The listing builds one solid part. Answer for the finished solid, in the listing's coordinates (mm). Face numbers are marked on the shaded views. Give positions to 0.01 mm unless a question says otherwise; leave off trailing zeros. Loops run counter-clockwise (first coordinate to the right, second up) from the corner with the lowest first, then second, coordinate; pieces in that order, holes last.
Item 1: The mould has two halves that part along Y. Classify the marked faces 1, 2, 3 and 4: pulls with the +Y half, pulls with the -Y half, needs draft (parallel to the pull), parting line crosses it, or undercut.
Item 2: Section B-B, the plane y = -11.5 is taken. Give the vertices of the cut face in (x, z) (1 decimal).
Item 3: Section D-D, the plane y = 7 is taken. Give the vertices of the cut face in (x, z) (3 decimals), and give its area (3 significant figures).
Item 4: Section C-C, the plane z = 6.25 is taken. Give the vertices of the cut face in (x, y) (3 decimals).
Item 5: Section A-A, the plane z = 3 is taken. Give the vertices of the cut face in (x, y) (3 decimals).
Item 6: This flat-tipped pin is pushed along its axis until it touches: pin 1 Ø5 at (x, y) = (-18.669, -12.319) entering from +Z (3 decimals). Where does it stop, or does it pass through?
Item 7: Consider line 1 along Y through (x, z) = (-13, 0.75) (3 decimals); line 2 along Y through (x, z) = (5, 1) (3 decimals); line 3 along Y through (x, z) = (19, 3.25) (3 decimals). Determine where each line is inside the solid, lowest interval first.
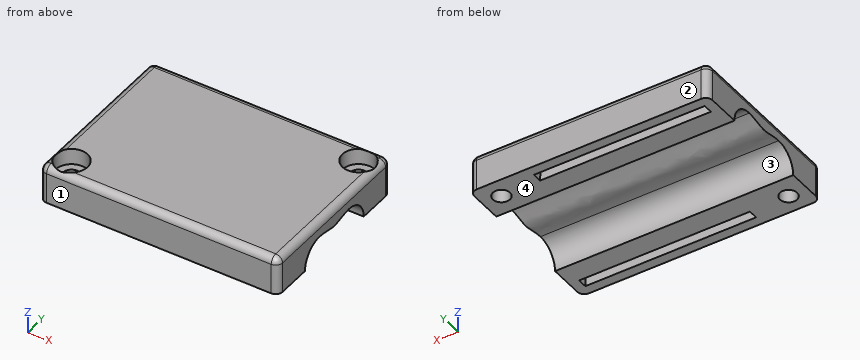
from build123d import *

# Parameters (mm, degrees)
F1_W          = 44.45
F1_H          = 31.75
F2_DEPTH      = 6.985
F4_DEPTH      = 44.45
F6_W          = 31.875
F6_H          = 1.75
F6_W_2        = 31.877
F7_DEPTH      = 2.5
F7_TAPER      = 7
F5_R          = 1.6
F8_DEPTH      = 25.4
F9_R          = 3
F9_R_2        = 1.6
F10_DEPTH     = 3
F11_T1_DEPTH  = 29.21
F11_T3_DEPTH  = 8.89
F11_T5_DEPTH  = 41.91
F11_S9_W      = 1.27
F11_S9_H      = 1.27
F11_T10_DEPTH = 1.27
F11_S15_W     = 1.27
F11_S15_H     = 1.27
F11_T16_DEPTH = 1.27
F11_S21_W     = 1.27
F11_S21_H     = 1.27
F11_T22_DEPTH = 1.27
F11_S27_W     = 1.27
F11_S27_H     = 1.27
F11_T28_DEPTH = 1.27


# Not quite as in the source:
# - a fillet or chamfer that OpenCascade refuses, or shapes differently, is made with other operations: its cross-section is extruded or revolved along the edge and cut away or added


with BuildPart() as f2:
    # F1 (on Top) → F2 (new body)
    with BuildSketch(Plane.XY):
        Rectangle(F1_W, F1_H)
    extrude(amount=F2_DEPTH)

    # F3 (on face) → F4 (cut, through all)
    with BuildSketch(Plane.YZ.offset(22.225)):
        with BuildLine():
            add(Edge.make_bspline(
                [(-4.125, 4.125), (-2.4255892558, 4.1137489608), (-0.0276085061, 2.971292738), (2.5249406681, 4.1137612248), (4.191, 4.191)],
                knots=[0, 0, 0, 0, 0.4977710734, 1, 1, 1, 1], degree=3))
            ThreePointArc((-4.125, 4.125), (-7.0418154724, 2.9168154724), (-8.25, 0))
            ThreePointArc((-8.25, 0), (-7.0418154724, -2.9168154724), (-4.125, -4.125))
            add(Edge.make_bspline(
                [(-4.125, -4.125), (-2.9335741419, -4.2006121948), (0.4172014685, -3.0581585459), (2.1438994445, -4.2006121948), (4.191, -4.191)],
                knots=[0, 0, 0, 0, 0.497799261, 1, 1, 1, 1], degree=3))
            ThreePointArc((4.191, -4.191), (7.15448452, -2.96348452), (8.382, 0))
            ThreePointArc((8.382, 0), (7.15448452, 2.96348452), (4.191, 4.191))
        make_face()
    extrude(amount=-F4_DEPTH, mode=Mode.SUBTRACT)

    # F6 (on Top) → F7 (cut)
    with BuildSketch(Plane.XY):
        with Locations((-4.4625, 13.175)):
            Rectangle(F6_W, F6_H)
        with Locations((4.4615, -13.175)):
            Rectangle(F6_W_2, F6_H)
    extrude(amount=F7_DEPTH, taper=F7_TAPER, mode=Mode.SUBTRACT)

    # F5 (on Top) → F8 (cut)
    with BuildSketch(Plane.XY):
        with Locations((-18.669, -12.319)):
            Circle(F5_R)
        with Locations((18.669, 12.319)):
            Circle(F5_R)
    extrude(amount=F8_DEPTH, mode=Mode.SUBTRACT)

    # F9 (on face) → F10 (cut)
    with BuildSketch(Plane.XY.offset(6.985)):
        with Locations((-18.669, -12.319)):
            Circle(F9_R)
        with Locations((-18.669, -12.319)):
            Circle(F9_R_2, mode=Mode.SUBTRACT)
        with Locations((18.669, 12.319)):
            Circle(F9_R)
        with Locations((18.669, 12.319)):
            Circle(F9_R_2, mode=Mode.SUBTRACT)
    extrude(amount=-F10_DEPTH, mode=Mode.SUBTRACT)

    # F11: fillet of radius 1.27 on 8 edges, made by hand

    # F11_s2 → F11_t1 (cut)
    with BuildSketch(Plane.XZ.offset(-14.605)):
        with BuildLine():
            ThreePointArc((-22.225, 5.715), (-21.8530256121, 6.6130256121), (-20.955, 6.985))
            Line((-20.955, 6.985), (-22.225, 6.985))
            Line((-22.225, 6.985), (-22.225, 5.715))
        make_face()
        with BuildLine():
            ThreePointArc((22.225, 5.715), (21.8530256121, 6.6130256121), (20.955, 6.985))
            Line((20.955, 6.985), (22.225, 6.985))
            Line((22.225, 6.985), (22.225, 5.715))
        make_face()
    extrude(amount=F11_T1_DEPTH, mode=Mode.SUBTRACT)

    # F11_s4 → F11_t3 (cut)
    with BuildSketch(Plane.XY.offset(-3.175)):
        with BuildLine():
            ThreePointArc((-22.225, -14.605), (-21.8530256121, -15.5030256121), (-20.955, -15.875))
            Line((-20.955, -15.875), (-22.225, -15.875))
            Line((-22.225, -15.875), (-22.225, -14.605))
        make_face()
        with BuildLine():
            ThreePointArc((22.225, -14.605), (21.8530256121, -15.5030256121), (20.955, -15.875))
            Line((20.955, -15.875), (22.225, -15.875))
            Line((22.225, -15.875), (22.225, -14.605))
        make_face()
        with BuildLine():
            ThreePointArc((20.955, 15.875), (21.8530256121, 15.5030256121), (22.225, 14.605))
            Line((22.225, 14.605), (22.225, 15.875))
            Line((22.225, 15.875), (20.955, 15.875))
        make_face()
        with BuildLine():
            ThreePointArc((-20.955, 15.875), (-21.8530256121, 15.5030256121), (-22.225, 14.605))
            Line((-22.225, 14.605), (-22.225, 15.875))
            Line((-22.225, 15.875), (-20.955, 15.875))
        make_face()
    extrude(amount=F11_T3_DEPTH, mode=Mode.SUBTRACT)

    # F11_s6 → F11_t5 (cut)
    with BuildSketch(Plane.YZ.offset(-20.955)):
        with BuildLine():
            ThreePointArc((-14.605, 6.985), (-15.5030256121, 6.6130256121), (-15.875, 5.715))
            Line((-15.875, 5.715), (-15.875, 6.985))
            Line((-15.875, 6.985), (-14.605, 6.985))
        make_face()
        with BuildLine():
            ThreePointArc((15.875, 5.715), (15.5030256121, 6.6130256121), (14.605, 6.985))
            Line((14.605, 6.985), (15.875, 6.985))
            Line((15.875, 6.985), (15.875, 5.715))
        make_face()
    extrude(amount=F11_T5_DEPTH, mode=Mode.SUBTRACT)


with BuildPart() as f11_tool8:
    # F11_s9 → F11_t10 (new body)
    with BuildSketch(Plane.XZ.offset(-14.605)):
        with Locations((-21.59, 6.35)):
            Rectangle(F11_S9_W, F11_S9_H)
    extrude(amount=-F11_T10_DEPTH)

    # F11_s11 → F11_t12 (revolve, cut)
    with BuildSketch(Plane(origin=(-20.955, 14.605, 5.715), x_dir=(0.7071067812, 0, -0.7071067812), z_dir=(0.7071067812, 0, 0.7071067812))):
        with BuildLine():
            ThreePointArc((0, -1.27), (1.27, 0), (0, 1.27))
            Line((0, 1.27), (0, -1.27))
        make_face()
    revolve(axis=Axis((-20.955, 14.605, 5.715), (0, 1, 0)), mode=Mode.SUBTRACT)


with BuildPart() as f2_1:
    add(f2.part)

    # F11_t7: cut F11_tool8
    add(f11_tool8.part, mode=Mode.SUBTRACT)


with BuildPart() as f11_tool14:
    # F11_s15 → F11_t16 (new body)
    with BuildSketch(Plane.XZ.offset(14.605)):
        with Locations((-21.59, 6.35)):
            Rectangle(F11_S15_W, F11_S15_H)
    extrude(amount=F11_T16_DEPTH)

    # F11_s17 → F11_t18 (revolve, cut)
    with BuildSketch(Plane(origin=(-20.955, -14.605, 5.715), x_dir=(0.7071067812, 0, -0.7071067812), z_dir=(-0.7071067812, 0, -0.7071067812))):
        with BuildLine():
            ThreePointArc((0, -1.27), (1.27, 0), (0, 1.27))
            Line((0, 1.27), (0, -1.27))
        make_face()
    revolve(axis=Axis((-20.955, -14.605, 5.715), (0, -1, 0)), mode=Mode.SUBTRACT)


with BuildPart() as f2_2:
    add(f2_1.part)

    # F11_t13: cut F11_tool14
    add(f11_tool14.part, mode=Mode.SUBTRACT)


with BuildPart() as f11_tool20:
    # F11_s21 → F11_t22 (new body)
    with BuildSketch(Plane.XZ.offset(14.605)):
        with Locations((21.59, 6.35)):
            Rectangle(F11_S21_W, F11_S21_H)
    extrude(amount=F11_T22_DEPTH)

    # F11_s23 → F11_t24 (revolve, cut)
    with BuildSketch(Plane(origin=(20.955, -14.605, 5.715), x_dir=(-0.7071067812, 0, -0.7071067812), z_dir=(-0.7071067812, 0, 0.7071067812))):
        with BuildLine():
            ThreePointArc((0, -1.27), (1.27, 0), (0, 1.27))
            Line((0, 1.27), (0, -1.27))
        make_face()
    revolve(axis=Axis((20.955, -14.605, 5.715), (0, -1, 0)), mode=Mode.SUBTRACT)


with BuildPart() as f2_3:
    add(f2_2.part)

    # F11_t19: cut F11_tool20
    add(f11_tool20.part, mode=Mode.SUBTRACT)


with BuildPart() as f11_tool26:
    # F11_s27 → F11_t28 (new body)
    with BuildSketch(Plane.XZ.offset(-14.605)):
        with Locations((21.59, 6.35)):
            Rectangle(F11_S27_W, F11_S27_H)
    extrude(amount=-F11_T28_DEPTH)

    # F11_s29 → F11_t30 (revolve, cut)
    with BuildSketch(Plane(origin=(20.955, 14.605, 5.715), x_dir=(-0.7071067812, 0, -0.7071067812), z_dir=(0.7071067812, 0, -0.7071067812))):
        with BuildLine():
            ThreePointArc((0, -1.27), (1.27, 0), (0, 1.27))
            Line((0, 1.27), (0, -1.27))
        make_face()
    revolve(axis=Axis((20.955, 14.605, 5.715), (0, 1, 0)), mode=Mode.SUBTRACT)


with BuildPart() as f2_4:
    add(f2_3.part)

    # F11_t25: cut F11_tool26
    add(f11_tool26.part, mode=Mode.SUBTRACT)


solid = f2_4.part
Worked answers:
1. face 1: pulls with the -Y half
1. face 2: pulls with the +Y half
1. face 3: undercut
1. face 4: needs draft
2. outline: (-22.2, 0) - (-20, 0) - (-20, 4) - (-21.6, 4) - (-21.6, 6.8) arc R1.3 ccw to (-22.2, 5.7) - close; (-17.3, 0) - (22.2, 0) - (22.2, 5.7) arc R1.3 ccw to (21, 7) - (-15.8, 7) - (-15.8, 4) - (-17.3, 4) - close
3. outline: (-22.225, 3.11) - (22.225, 3.11) - (22.225, 5.715) arc R1.27 ccw to (20.955, 6.985) - (-20.955, 6.985) arc R1.27 ccw to (-22.225, 5.715) - close
3. area: 172 mm2
4. outline: (-22.107, -14.605) arc R1.152 ccw to (-20.955, -15.757) - (20.955, -15.757) arc R1.152 ccw to (22.107, -14.605) - (22.107, 14.605) arc R1.152 ccw to (20.955, 15.757) - (-20.955, 15.757) arc R1.152 ccw to (-22.107, 14.605) - close; hole circle Ø6 at (-18.669, -12.319); hole circle Ø6 at (18.669, 12.319)
5. outline: (-22.225, -14.605) arc R1.27 ccw to (-20.955, -15.875) - (20.955, -15.875) arc R1.27 ccw to (22.225, -14.605) - (22.225, -6.956) - (-22.225, -6.956) - close; (-22.225, 7.118) - (22.225, 7.118) - (22.225, 14.605) arc R1.27 ccw to (20.955, 15.875) - (-20.955, 15.875) arc R1.27 ccw to (-22.225, 14.605) - close; hole circle Ø3.2 at (-18.669, -12.319); hole circle Ø3.2 at (18.669, 12.319)
6. pin 1: stops at z = 3.985
7. line 1: y = -15.875 to -8.181, 8.314 to 12.392, 13.958 to 15.875
7. line 2: y = -15.875 to -13.927, -12.423 to -8.127, 8.261 to 12.423, 13.927 to 15.875
7. line 3: y = -15.875 to -6.665, 6.837 to 10.754, 13.884 to 15.875
